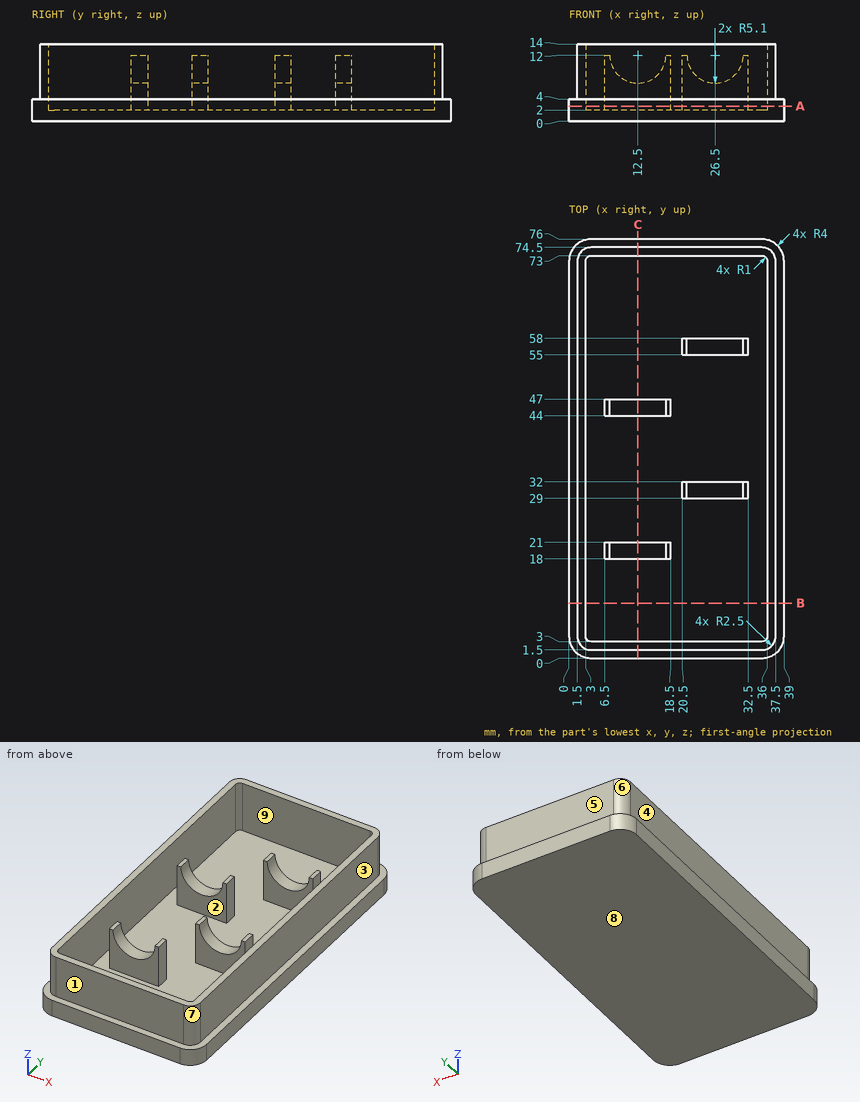
Part print with two shaded views. Sizes in mm from the minimum x, y, z corner. A direction names the side the tool comes from. Round coordinates to 2 decimals unless told otherwise and drop trailing zeros. Order: outer loops, then holes, each group sorted by start corner. A loop starts at its lowest first (then second) coordinate and runs counter-clockwise, first axis right, second up. Notation, with made-up numbers: (66, 15) - (86, 15) arc R30 ccw to (86, 39) - close; hole circle Ø5 at (-22, 70). An arc over 180 degrees is marked (long way). Return JSON: item names as keys, results as strings.
(1) Cut at A-A (z = 2.75). State how many separate pieces and enclosed holes the cut face has, then the cut area to 3 significant figures.
Answer key:
{"separate pieces": "5", "enclosed holes": "1", "area": "785 mm^2"}
(2) Cut at C-C (x = 12.5). Give the cut face in (y, z), then the cut area to 3 significant figures.
Answer key:
{"outline": "(0, 0) - (76, 0) - (76, 4) - (74.5, 4) - (74.5, 14) - (73, 14) - (73, 2) - (47, 2) - (47, 6.9) - (44, 6.9) - (44, 2) - (21, 2) - (21, 6.9) - (18, 6.9) - (18, 2) - (3, 2) - (3, 14) - (1.5, 14) - (1.5, 4) - (0, 4) - close", "area": "223 mm^2"}
(3) Tool access for the marked faces 1, 2, 3, 4 and 5: list every direction of +Z, -Z, +X, -X, +Y, -Y with a clear straight run to the whole face (end or side of a thin tool).
Answer key:
{"face 1": "+Z, +X, -X, -Y", "face 2": "+Z", "face 3": "+Z, +X, +Y, -Y", "face 4": "+Z, -X, +Y, -Y", "face 5": "+Z, +X, -X, +Y"}
(4) Cut at B-B (y = 10). Give the cut face in (x, z).
Answer key:
{"outline": "(0, 0) - (39, 0) - (39, 4) - (37.5, 4) - (37.5, 14) - (36, 14) - (36, 2) - (3, 2) - (3, 14) - (1.5, 14) - (1.5, 4) - (0, 4) - close"}
(5) Pull direction X, two halves, no side cores. Call the marked faces 6, 7, 8 and 9: +X half, -X half, draft (parallel to the pull), parting line (faces both ways), or undercut.
Answer key:
{"face 6": "-X half", "face 7": "+X half", "face 8": "draft", "face 9": "undercut"}
(6) Pin check, flat tips, straight feed: pin 1 Ø3 at (x, z) = (13.5, 8) entering from +Y; pin 2 Ø3 at (x, z) = (25.5, 9.5) entering from -Y; pin 3 Ø12 at (x, y) = (16.5, 51) entering from +Z. Stop position of each tip, or through.
Answer key:
{"pin 1": "stops at y = 74.5", "pin 2": "stops at y = 1.5", "pin 3": "stops at z = 12"}
(7) Wall check: probe 1 along Y at (x, z) = (11, 3.5); probe 2 along Y at (x, z) = (29, 2.5); probe 3 along X at (y, z) = (22.5, 3). Give the ranges that are in metal, low to high. Write a range as from..to.
Answer key:
{"probe 1": "y = 0..3, 18..21, 44..47, 73..76", "probe 2": "y = 0..3, 29..32, 55..58, 73..76", "probe 3": "x = 0..3, 36..39"}
